Autodesk Inventor part; units mm, degrees
ref_plane "YZ Plane" through (0, 0, 0) normal (1, 0, 0) x (0, 1, 0)
ref_plane "XZ Plane" through (0, 0, 0) normal (0, 1, 0) x (-1, 0, 0)
ref_plane "XY Plane" through (0, 0, 0) normal (0, 0, 1) x (1, 0, 0)
sketch "Sketch1" plane through (0, 0, 0) normal (0, 1, 0) x (-1, 0, 0)
  line L0 (30.85, -12.5) -> (30.85, 12.5)
  line L1 (30.85, 12.5) -> (0, 18)
  line L2 (0, 18) -> (-30.85, 12.5)
  line L3 (-30.85, 12.5) -> (-30.85, -12.5)
  line L4 (-30.85, -12.5) -> (0, -18)
  line L5 (0, -18) -> (30.85, -12.5)
  point P0 (0, 0)
  point P1 (30.85, 0)
  point P2 (-30.85, 0)
  dimension "d0" = 61.7
  dimension "d1" = 25
  dimension "d2" = 36
extrude "Extrusion1" add sketch "Sketch1" along normal mid plane 1.7
properties part number "Speaker" material "Paper"
Read the model definition and answer for the solid it produces. Units are mm, in the model's axes. Give positions to 0.01 mm unless a question says otherwise; leave off trailing zeros. Write each loop counter-clockwise with the first axis right and the second up, starting at its lowest first coordinate (ties: lowest second). Pieces come first, ordered by that corner, then holes. Notation, with made-up numbers: (5.5, 12) -> (10.5, 12) arc R18 ccw to (10.5, 17) -> close; hole circle Ø3 at (84, 37). An arc over 180 degrees is marked (long way). Answer as a JSON object with one key per item and string values.
1) Straight lines are drawn through the part: probe 1 along Z at (x, y) = (-10, 0); probe 2 along Z at (x, y) = (-15.5, -0.3). For each, find the intervals that lie inside material, in ascending order. Write a range as from..to.
Findings below:
{"probe 1": "z = -16.22..16.22", "probe 2": "z = -15.24..15.24"}
2) Section A-A on y = 0.15 is taken. Write down the section's boundary in (x, z), then the cut area to 3 significant figures.
Findings below:
{"outline": "(-30.85, -12.5) -> (0, -18) -> (30.85, -12.5) -> (30.85, 12.5) -> (0, 18) -> (-30.85, 12.5) -> close", "area": "1,880 mm^2"}
3) Section C-C on z = -15 is taken. Write down the section's boundary in (x, y).
Findings below:
{"outline": "(-16.83, -0.85) -> (16.83, -0.85) -> (16.83, 0.85) -> (-16.83, 0.85) -> close"}
4) Section B-B on x = 21 is taken. Write down the section's boundary in (y, z), then the cut area to 3 significant figures.
Findings below:
{"outline": "(-0.85, -14.26) -> (0.85, -14.26) -> (0.85, 14.26) -> (-0.85, 14.26) -> close", "area": "48.5 mm^2"}
5) A flat-ended cylindrical pin translates along its axis: pin 1 Ø1 at (x, y) = (-24.5, 0) entering from +Z. Find the tip coordinate at first contact, or state that the pin passes through.
Findings below:
{"pin 1": "stops at z = 13.72"}
